from build123d import *

# Parameters (mm, degrees)
SKETCH_2_R          = 1.5
EXTRUDE_1_DEPTH     = 27
SHELL_1_DEPTH       = 24
CUT_EXTRUDE_START   = -24
SKETCH_3_R          = 3
CUT_EXTRUDE_1_DEPTH = 24
SKETCH_5_W          = 20
SKETCH_5_H          = 6
CUT_EXTRUDE_3_DEPTH = 32
SKETCH_6_W          = 4
SKETCH_6_H          = 12
CUT_EXTRUDE_4_DEPTH = 32
SKETCH_7_W          = 10
SKETCH_7_H          = 8
CUT_EXTRUDE_5_DEPTH = 32
EXTRUDE_2_DEPTH     = 24
SKETCH_9_W          = 10
SKETCH_9_H          = 3
CUT_EXTRUDE_6_DEPTH = 24
SKETCH_10_R         = 1.35
CUT_EXTRUDE_7_DEPTH = 10
CUT_EXTRUDE_8_DEPTH = 10
CUT_EXTRUDE_9_DEPTH = 10


# Read off the part's stored shape, not the designer's step: 抽壳1
with BuildPart() as part:
    # 草图2 → 凸台-拉伸1 (new body)
    with BuildSketch(Plane.XY):
        with BuildLine():
            Line((-76.5, 30.151923789), (-76.5, -30.151923789))
            ThreePointArc((-76.5, -30.151923789), (-77.380060021, -34.576284287), (-72.878679656, -34.871320344))
            Line((-72.878679656, -34.871320344), (-57.32, -50.43))
            Line((-57.32, -50.43), (57.32, -50.43))
            Line((57.32, -50.43), (72.878679656, -34.871320344))
            ThreePointArc((72.878679656, -34.871320344), (77.380060021, -34.576284287), (76.5, -30.151923789))
            Line((76.5, -30.151923789), (76.5, 30.151923789))
            ThreePointArc((76.5, 30.151923789), (77.593259199, 34.258312544), (73.483390382, 35.33841559))
            Line((73.483390382, 35.33841559), (40.238526366, 54.25))
            Line((40.238526366, 54.25), (-40.760907637, 54.25))
            Line((-40.760907637, 54.25), (-73.5, 35.348076211))
            ThreePointArc((-73.5, 35.348076211), (-77.598076211, 34.25), (-76.5, 30.151923789))
        make_face()
        with Locations((-75, 32.75)):
            Circle(SKETCH_2_R, mode=Mode.SUBTRACT)
        with Locations((75, 32.75)):
            Circle(SKETCH_2_R, mode=Mode.SUBTRACT)
        with Locations((75, -32.75)):
            Circle(SKETCH_2_R, mode=Mode.SUBTRACT)
        with Locations((-75, -32.75)):
            Circle(SKETCH_2_R, mode=Mode.SUBTRACT)
    extrude(amount=EXTRUDE_1_DEPTH)

    # 抽壳1 outline → 抽壳1 (cut)
    with BuildSketch(Plane.XY):
        with BuildLine():
            Line((-73.5, 28.507359313), (-73.5, -28.507359313))
            ThreePointArc((-73.5, -28.507359313), (-71.254879923, -30.255190266), (-70.506971411, -33.000387902))
            Line((-70.506971411, -33.000387902), (-56.077359313, -47.43))
            Line((-56.077359313, -47.43), (56.077359313, -47.43))
            Line((56.077359313, -47.43), (70.506971411, -33.000387902))
            ThreePointArc((70.506971411, -33.000387902), (71.254879923, -30.255190266), (73.5, -28.507359313))
            Line((73.5, -28.507359313), (73.5, 28.507359313))
            ThreePointArc((73.5, 28.507359313), (71.110106029, 30.48754008), (70.570593139, 33.543948905))
            Line((70.570593139, 33.543948905), (39.444948236, 51.25))
            Line((39.444948236, 51.25), (-39.95706006, 51.25))
            Line((-39.95706006, 51.25), (-70.575765386, 33.572282238))
            ThreePointArc((-70.575765386, 33.572282238), (-71.102885683, 30.5), (-73.5, 28.507359313))
        make_face()
    extrude(amount=SHELL_1_DEPTH, mode=Mode.SUBTRACT)

    # 草图3 → 切除-拉伸1 (cut)
    with BuildSketch(Plane.XY.offset(27).offset(CUT_EXTRUDE_START)):
        with Locations((75, 32.75)):
            Circle(SKETCH_3_R)
        with Locations((75, -32.75)):
            Circle(SKETCH_3_R)
        with Locations((-75, -32.75)):
            Circle(SKETCH_3_R)
        with Locations((-75, 32.75)):
            Circle(SKETCH_3_R)
    extrude(amount=CUT_EXTRUDE_1_DEPTH, mode=Mode.SUBTRACT)

    # 草图5 → 切除-拉伸3 (cut)
    with BuildSketch(Plane.XY.offset(27)):
        with Locations((20.7074416, -19.577067137)):
            Rectangle(SKETCH_5_W, SKETCH_5_H)
    extrude(amount=-CUT_EXTRUDE_3_DEPTH, mode=Mode.SUBTRACT)

    # 草图6 → 切除-拉伸4 (cut)
    with BuildSketch(Plane(origin=(76.5, 0, 0), x_dir=(0, 0, -1), z_dir=(1, 0, 0))):
        with Locations((-2, 20.977362477)):
            Rectangle(SKETCH_6_W, SKETCH_6_H)
    extrude(amount=-CUT_EXTRUDE_4_DEPTH, mode=Mode.SUBTRACT)

    # 草图7 → 切除-拉伸5 (cut)
    with BuildSketch(Plane(origin=(33.153284591, 58.280491682, 0), x_dir=(0.8692042501767389, -0.4944532045347601, 0), z_dir=(0.4944532045347601, 0.8692042501767389, 0))):
        with Locations((38.03253292, -4)):
            Rectangle(SKETCH_7_W, SKETCH_7_H)
    extrude(amount=-CUT_EXTRUDE_5_DEPTH, mode=Mode.SUBTRACT)

    # 草图8 → 凸台-拉伸2 (add)
    with BuildSketch(Plane.XY.offset(27)):
        Polygon((40.238526366, 54.25), (40.238526366, 62.25), (15.238526366, 62.25), (15.238526366, 54.25), (17.238526366, 54.25), (17.238526366, 60.25), (38.238526366, 60.25), (38.238526366, 54.25), align=None)
    extrude(amount=-EXTRUDE_2_DEPTH)

    # 草图9 → 切除-拉伸6 (cut)
    with BuildSketch(Plane(origin=(0, 54.25, 0), x_dir=(1, 0, 0), z_dir=(0, 1, 0))):
        with Locations((27.738526366, -1.5)):
            Rectangle(SKETCH_9_W, SKETCH_9_H)
    extrude(amount=-CUT_EXTRUDE_6_DEPTH, mode=Mode.SUBTRACT)

    # 草图10 → 切除-拉伸7 (cut)
    with BuildSketch(Plane.XZ.offset(50.43)):
        with Locations((-18.75, 20)):
            Circle(SKETCH_10_R)
        with Locations((18.75, 20)):
            Circle(SKETCH_10_R)
    extrude(amount=-CUT_EXTRUDE_7_DEPTH, mode=Mode.SUBTRACT)

    # 草图11 → 切除-拉伸8 (cut)
    with BuildSketch(Plane.XZ.offset(50.43)):
        Polygon((0, 3), (2, 3), (2, 0), (-2, 0), (-2, 3), align=None)
    extrude(amount=-CUT_EXTRUDE_8_DEPTH, mode=Mode.SUBTRACT)

    # 草图12 → 切除-拉伸9 (cut)
    with BuildSketch(Plane.XZ.offset(50.43)):
        Polygon((-24.75, 20), (-24.75, 27), (24.75, 27), (24.75, 20), (24.75, 0), (-24.75, 0), align=None)
    extrude(amount=-CUT_EXTRUDE_9_DEPTH, mode=Mode.SUBTRACT)


solid = part.part
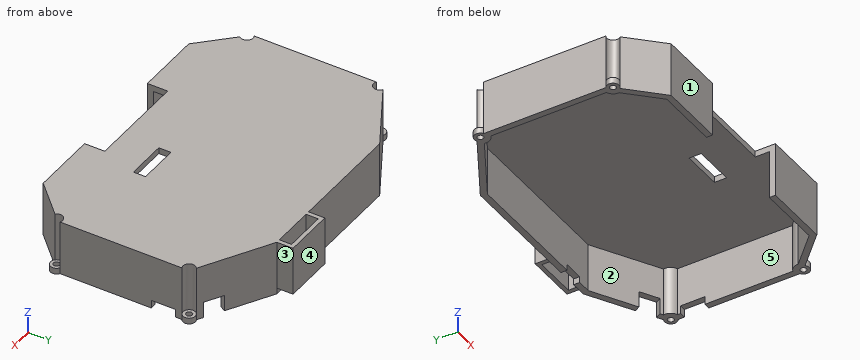
Build history of the part. All positions in model axes, mm. Face numbers are marked on the shaded views. A direction names the side the tool comes from. Round coordinates to 2 decimals unless told otherwise and drop trailing zeros. Write each loop counter-clockwise with the first axis right and the second up, starting at its lowest first coordinate (ties: lowest second). Pieces come first, ordered by that corner, then holes. Notation, with made-up numbers: M -33.75,36 L 9.25,36 A22 cw 9.25,62 Z; hole C 57,8.5 d4. An arc over 180 degrees is marked long. Answer as a JSON object with one key per item and string values. Group by question number.
(1) Cut at C-C (x = 6.5). Give the cut face in (y, z).
(2) Drill centre lines: L1, parallel to Y at x = -75, z = 0.7; L2, parallel to X at y = -32.75, z = 1.85; L3, parallel to Y at x = 75, z = 1.2. Where is each one in solid material? Low to high.
(3) Flat gauge pins, fed straight in: pin 1 (3.5 mm diameter, centred on y = 52, z = 1.5, fed in from -X); pin 2 (6 mm diameter, centred on x = 67.5, y = 39.5, fed in from -Z); pin 3 (10 mm diameter, centred on x = -19.5, z = 6, fed in from +Y). Where does each tip first touch, or does it go through?
(4) Mould opens along X. For the marked faces 1, 2 and 3 say: pulls with the +X half, pulls with the -X half, needs draft (parallel to the pull), parting line crosses it, or undercut.
(5) Cut at A-A (x = -32.5). Give the cut face in (y, z).
(6) Cut at B-B (y = -26). Give the cut face in (x, z), and give its area (3 significant figures).
(7) Which spindle directions (+Z, -Z, +X, -X, +Y, -Y) get a long thin tool onto all of the face, cutting with end or side? Do the marked faces 4 and 5. Say none if no direction does.
Responses:
{
 "1": {"outline": "M -40.43,24 L 51.25,24 L 51.25,0 L 54.25,0 L 54.25,27 L -40.43,27 Z"},
 "2": {"L1": "y = -35.75 to -34.25, -31.25 to 31.25, 34.25 to 35.75", "L2": "x = -78 to -76.5, -73.5 to -70.5, 70.5 to 73.5, 76.5 to 78", "L3": "y = -35.75 to -34.25, -31.25 to 14.98, 26.98 to 31.25, 34.25 to 35.75"},
 "3": {"pin 1": "stops at x = -47.69", "pin 2": "stops at z = 8", "pin 3": "stops at y = 54.25"},
 "4": {"face 1": "needs draft", "face 2": "undercut", "face 3": "pulls with the +X half"},
 "5": {"outline": "M -50.43,0 L -47.43,0 L -47.43,24 L 51.25,24 L 51.25,0 L 54.25,0 L 54.25,27 L -50.43,27 Z"},
 "6": {"outline": "M -76.5,0 L -73.5,0 L -73.5,24 L 73.5,24 L 73.5,0 L 76.5,0 L 76.5,27 L -76.5,27 Z", "area": "603 mm2"},
 "7": {"face 4": "+Z, -Z, +X, -X, +Y", "face 5": "-Z"}
}
